Here's the drawing with two shaded views (mm, measured from the low corner). I have some questions. A direction names the side the tool comes from. Coordinates: 2 decimals unless noted, no trailing zeros. Loops run counter-clockwise (first coordinate to the right, second up) from the corner with the lowest first, then second, coordinate; pieces in that order, holes last. Notation, with made-up numbers: (-14, 22) - (-9, 22) arc R24 cw to (-9, 56) - close; hole circle Ø11 at (25, -13). An arc over 180 degrees is marked (long way). Use a Markdown table: item, result.
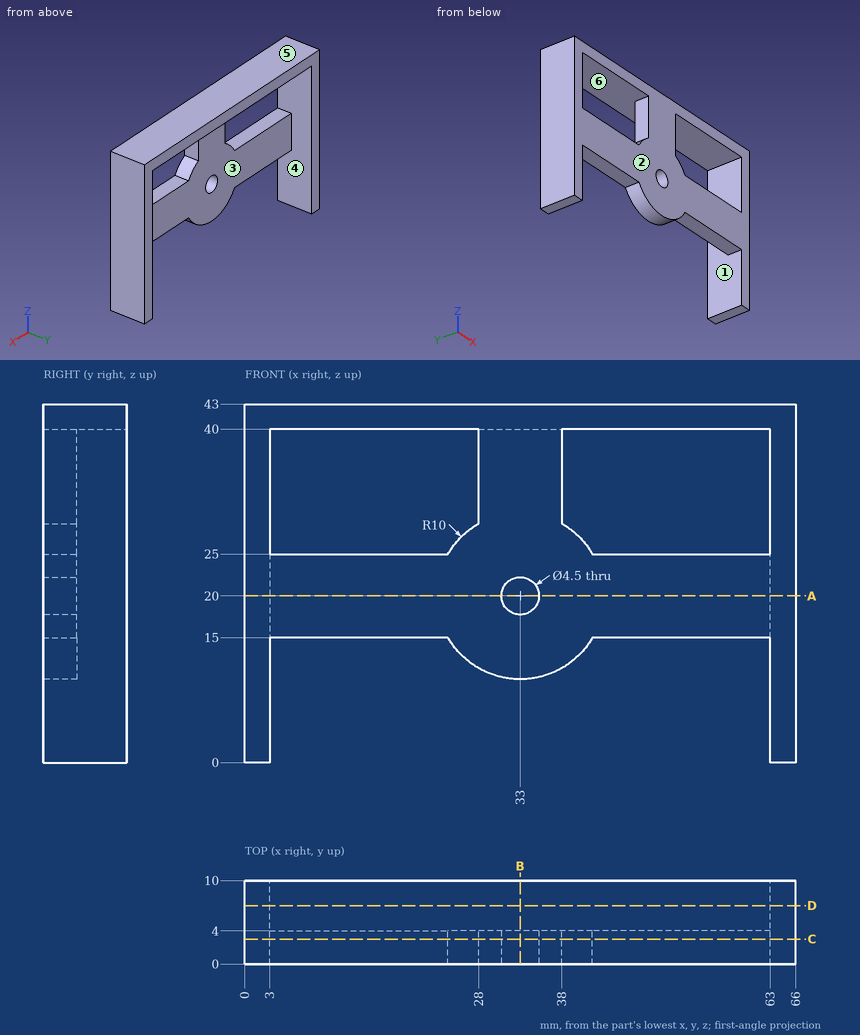
Q1. Please list where these lines run through material, in increasing order: L1, parallel to X at y = 1, z = 38; L2, parallel to X at y = 2.1, z = 20; L3, parallel to X at y = 6.75, z = 31. Write a range as from..to.
Check values:
| item | result |
|---|---|
| L1 | 0..3, 28..38, 63..66 |
| L2 | 0..30.75, 35.25..66 |
| L3 | 0..3, 63..66 |
Q2. I want a section at D-D, the plane y = 7. Write out the boundary of the cut face in (x, z).
Check values:
| item | result |
|---|---|
| outline | (0, 0) - (3, 0) - (3, 40) - (63, 40) - (63, 0) - (66, 0) - (66, 43) - (0, 43) - close |
Q3. Will these pins go through, and if not, where does the flat tip stop? P1, Ø1.2, axis at x = 47, y = 2.5, coming from the -Z side; P2, Ø9, axis at x = 42, z = 24, coming from the +Y side; P3, Ø6, axis at x = 25.5, y = 4, coming from the -Z side.
Check values:
| item | result |
|---|---|
| P1 | z = 15 |
| P2 | y = 4 |
| P3 | z = 11.07 |
Q4. If we mould it in two halves opening along Z, with no side actions, what happens to the marked faces 3, 4, 5 and 6? For each: pulls with the +Z half, pulls with the -Z half, needs draft (parallel to the pull), parting line crosses it, or undercut.
Check values:
| item | result |
|---|---|
| face 3 | needs draft |
| face 4 | undercut |
| face 5 | pulls with the +Z half |
| face 6 | undercut |
Q5. I want a section at A-A, the plane z = 20. Write out the boundary of the cut face in (x, y), then the cut area to 3 significant figures.
Check values:
| item | result |
|---|---|
| outline | (0, 0) - (30.75, 0) - (30.75, 4) - (3, 4) - (3, 10) - (0, 10) - close; (35.25, 0) - (66, 0) - (66, 10) - (63, 10) - (63, 4) - (35.25, 4) - close |
| area | 282 mm^2 |
Q6. Which directions (+Z, -Z, +X, -X, +Y, -Y) give clear straight access to the entire face, cutting with the end or side of a thin tool? Please do the marked faces 1 and 2.
Check values:
| item | result |
|---|---|
| face 1 | +Y |
| face 2 | +Z, -Z, +X, -X, -Y |
Q7. I want a section at B-B, the plane x = 33. Write out the boundary of the cut face in (y, z).
Check values:
| item | result |
|---|---|
| outline | (0, 10) - (4, 10) - (4, 17.75) - (0, 17.75) - close; (0, 22.25) - (4, 22.25) - (4, 40) - (10, 40) - (10, 43) - (0, 43) - close |
Q8. I want a section at C-C, the plane y = 3. Write out the boundary of the cut face in (x, z).
Check values:
| item | result |
|---|---|
| outline | (0, 0) - (3, 0) - (3, 15) - (24.34, 15) arc R10 ccw to (41.66, 15) - (63, 15) - (63, 0) - (66, 0) - (66, 43) - (0, 43) - close; hole (3, 25) - (24.34, 25) arc R10 cw to (28, 28.66) - (28, 40) - (3, 40) - close; hole circle Ø4.5 at (33, 20); hole (38, 28.66) arc R10 cw to (41.66, 25) - (63, 25) - (63, 40) - (38, 40) - close |
